For this review, take the finished solid that the model builds, in its own axes (mm). A direction names the side the tool comes from. Give positions to 0.01 mm unless a question says otherwise; leave off trailing zeros. Write each loop counter-clockwise with the first axis right and the second up, starting at its lowest first coordinate (ties: lowest second). Pieces come first, ordered by that corner, then holes.
1) Machinability: for faces 4 (the face through (15.365, 0.021, -16.809)), 5 (the face through (-7, 0, 30)), which of the approach directions +Z, -Z, +X, -X, +Y, -Y give a long, thin tool a straight path to every point of the face, cutting with its end or side? Answer none if there is none.
2) Wall thickness on line 1 along X through (y, z) = (0.7, 8); line 2 along X through (y, z) = (-0.6, 5.5); line 3 along Z through (x, y) = (16.5, 0.65): over which ranges is each line inside the solid? List them lowest first.
3) We need section D-D on z = 5. Give the boundary of the cut face in (x, y), and give its area (3 significant figures).
4) For P1, Ø3, axis at x = 17.9, z = -34, coming from the +Y side, flat-tipped, find the tip position at first contact; note if it passes through.
5) We need section C-C on x = -21. Give the boundary of the cut face in (y, z), and give its area (3 significant figures).
6) We need section B-B on x = 6. Give the boundary of the cut face in (y, z), and give its area (3 significant figures).
7) Draft analysis for pull direction X (two halves, no side actions). For faces 1 (the face through (-30, 0, -7)), 2 (the face through (18.275, -0.021, -42.295)), 3 (the face through (-19, 0, 0)), state which applies: pulls with the +X half, pulls with the -X half, needs draft (parallel to the pull), parting line crosses it, or undercut.
8) We need section A-A on z = 25. Give the boundary of the cut face in (x, y).
from build123d import *

# Parameters (mm, degrees)
SKETCH_4_R          = 1.6
EXTRUDE_1_DEPTH     = 1.5
CUT_EXTRUDE_2_DEPTH = 3
FILLET_2_R          = 1.75


with BuildPart() as part:
    # ｽｹｯﾁ4 → ﾎﾞｽ - 押し出し1 (new, symmetric)
    with BuildSketch(Plane(origin=(0, 0, 0), x_dir=(1, 0, 0), z_dir=(0, 1, 0))):
        Polygon((-30, 0), (-30, 15), (18.480762114, 42.990381057), (25.980762114, 30), (0, -30), (-15, -30), align=None)
        with Locations(Location((0.580127019, 23.995190528, 0), (0, 0, 270))):
            Circle(SKETCH_4_R, mode=Mode.SUBTRACT)
        with Locations(Location((-5, 7.5, 0), (0, 0, 270))):
            Circle(SKETCH_4_R, mode=Mode.SUBTRACT)
        with Locations(Location((-7.5, -5, 0), (0, 0, 270))):
            Circle(SKETCH_4_R, mode=Mode.SUBTRACT)
        with Locations(Location((-7.5, -25, 0), (0, 0, 270))):
            Circle(SKETCH_4_R, mode=Mode.SUBTRACT)
        with Locations(Location((-25, 7.5, 0), (0, 0, 270))):
            Circle(SKETCH_4_R, mode=Mode.SUBTRACT)
        with Locations(Location((17.900635095, 33.995190528, 0), (0, 0, 270))):
            Circle(SKETCH_4_R, mode=Mode.SUBTRACT)
    extrude(amount=EXTRUDE_1_DEPTH, both=True)

    # ｽｹｯﾁ5 → ｶｯﾄ - 押し出し2 (cut)
    with BuildSketch(Plane(origin=(0, 1.5, 0), x_dir=(1, 0, 0), z_dir=(0, 1, 0))):
        Polygon((12.665448219, 10.574351407), (19.442413698, 26.225082782), (6.92820323, 19), (4.714101615, 15.165063509), align=None)
        Polygon((4.714101615, 15.165063509), (6.92820323, 19), (2.5, 16.443375673), align=None)
        Polygon((2.214101615, 10.834936491), (0, 12.113248654), (0, 7), align=None)
        Polygon((0, 0), (0, -18.675248347), (10.665448219, 5.955549254), (2.214101615, 10.834936491), (0, 7), align=None)
        Polygon((-15, 0), (-24.968847051, 0), (-15, -19.937694101), align=None)
    extrude(amount=-CUT_EXTRUDE_2_DEPTH, mode=Mode.SUBTRACT)

    # ﾌｨﾚｯﾄ2
    fillet_2_edges = [part.edges().sort_by_distance(p)[0] for p in [
        (-30, 0, 0),
        (-30, 0, -15),
        (18.480762114, 0, -42.990381057),
        (25.980762114, 0, -30),
        (0, 0, 30),
        (-15, 0, 30),
        (-24.968847051, 0, 0),
        (-15, 0, 0),
        (-15, 0, 19.937694101),
        (0, 0, 18.675248347),
        (0, 0, -12.113248654),
        (10.665448219, 0, -5.955549254),
        (2.5, 0, -16.443375673),
        (19.442413698, 0, -26.225082782),
        (12.665448219, 0, -10.574351407),
    ]]
    fillet(fillet_2_edges, radius=FILLET_2_R)


solid = part.part
Results list:
1. face 4: +Y, -Y
1. face 5: +Z, +X, -X, +Y, -Y
2. line 1: x = -26 to -20.97, -15 to 0, 4.62 to 9.53
2. line 2: x = -27.25 to -22.22, -15 to -9.02, -5.98 to 0, 5.71 to 10.61
2. line 3: z = -41.85 to -34.77, -33.22 to -23.64, -19.43 to -8.11
3. outline: (-27.5, -1.5) - (-22.47, -1.5) - (-22.47, 1.5) - (-27.5, 1.5) - close; (-15, -1.5) - (-9.1, -1.5) - (-9.1, 1.5) - (-15, 1.5) - close; (-5.9, -1.5) - (0, -1.5) - (0, 1.5) - (-5.9, 1.5) - close; (5.92, -1.5) - (10.83, -1.5) - (10.83, 1.5) - (5.92, 1.5) - close
3. area: 65.2 mm2
4. P1: passes through
5. outline: (-1.5, -20.2) - (1.5, -20.2) - (1.5, 0) - (-1.5, 0) - close; (-1.5, 7.94) - (1.5, 7.94) - (1.5, 18) - (-1.5, 18) - close
5. area: 90.8 mm2
6. outline: (-1.5, -35.78) - (1.5, -35.78) - (1.5, -18.46) - (-1.5, -18.46) - close; (-1.5, -14.42) - (1.5, -14.42) - (1.5, -8.65) - (-1.5, -8.65) - close; (-1.5, 4.82) - (1.5, 4.82) - (1.5, 16.14) - (-1.5, 16.14) - close
6. area: 103 mm2
7. face 1: pulls with the -X half
7. face 2: parting line crosses it
7. face 3: undercut
8. outline: (-17.5, -1.5) - (-9.1, -1.5) - (-9.1, 1.5) - (-17.5, 1.5) - close; (-5.9, -1.5) - (2.17, -1.5) - (2.17, 1.5) - (-5.9, 1.5) - close
